from build123d import *

# Parameters (mm, degrees)
EXTRUDE_1_DEPTH     = 1300
SKETCH_3_R          = 2
CUT_EXTRUDE_1_DEPTH = 1301.046633779
CUT_EXTRUDE_2_DEPTH = 1500
SKETCH_5_R          = 2
CUT_EXTRUDE_3_DEPTH = 1301.046633779


with BuildPart() as part:
    # 草图2 → 凸台-拉伸1 (new body)
    with BuildSketch(Plane.XY):
        with BuildLine():
            Line((-0.5, 8.5), (0.5, 8.5))
            ThreePointArc((0.5, 8.5), (2.621320344, 7.621320344), (3.5, 5.5))
            Line((3.5, 5.5), (3.5, -5.5))
            ThreePointArc((3.5, -5.5), (2.621320344, -7.621320344), (0.5, -8.5))
            Line((0.5, -8.5), (-0.5, -8.5))
            ThreePointArc((-0.5, -8.5), (-2.621320344, -7.621320344), (-3.5, -5.5))
            Line((-3.5, -5.5), (-3.5, 5.5))
            ThreePointArc((-3.5, 5.5), (-2.621320344, 7.621320344), (-0.5, 8.5))
        make_face()
    extrude(amount=EXTRUDE_1_DEPTH)

    # 草图3 → 切除-拉伸1 (cut, through all)
    with BuildSketch(Plane.ZY.offset(3.5)):
        with Locations((100, 0)):
            Circle(SKETCH_3_R)
        with Locations((200, 0)):
            Circle(SKETCH_3_R)
        with Locations((300, 0)):
            Circle(SKETCH_3_R)
        with Locations((400, 0)):
            Circle(SKETCH_3_R)
        with Locations((500, 0)):
            Circle(SKETCH_3_R)
        with Locations((600, 0)):
            Circle(SKETCH_3_R)
        with Locations((700, 0)):
            Circle(SKETCH_3_R)
        with Locations((800, 0)):
            Circle(SKETCH_3_R)
        with Locations((900, 0)):
            Circle(SKETCH_3_R)
        with Locations((1000, 0)):
            Circle(SKETCH_3_R)
    extrude(amount=-CUT_EXTRUDE_1_DEPTH, mode=Mode.SUBTRACT)

    # 草图4 → 切除-拉伸2 (cut)
    with BuildSketch(Plane(origin=(0, 0, 0), x_dir=(-1, 0, 0), z_dir=(0, 0, -1))):
        with BuildLine():
            Line((-0.5, 7), (0.5, 7))
            ThreePointArc((0.5, 7), (1.560660172, 6.560660172), (2, 5.5))
            Line((2, 5.5), (2, -5.90279402))
            ThreePointArc((2, -5.90279402), (1.678635809, -6.678635809), (0.90279402, -7))
            Line((0.90279402, -7), (-0.90279402, -7))
            ThreePointArc((-0.90279402, -7), (-1.678635809, -6.678635809), (-2, -5.90279402))
            Line((-2, -5.90279402), (-2, 5.5))
            ThreePointArc((-2, 5.5), (-1.560660172, 6.560660172), (-0.5, 7))
        make_face()
    extrude(amount=-CUT_EXTRUDE_2_DEPTH, mode=Mode.SUBTRACT)

    # 草图5 → 切除-拉伸3 (cut, through all)
    with BuildSketch(Plane.ZY.offset(3.5)):
        with Locations((1100, 0)):
            Circle(SKETCH_5_R)
        with Locations((1200, 0)):
            Circle(SKETCH_5_R)
        with Locations((1250, 0)):
            Circle(SKETCH_5_R)
        with Locations((1150, 0)):
            Circle(SKETCH_5_R)
    extrude(amount=-CUT_EXTRUDE_3_DEPTH, mode=Mode.SUBTRACT)


solid = part.part
Input: part model. Units: mm. Frame: model coordinates. Give positions to 0.01 mm unless a question says otherwise; leave off trailing zeros. Order: outer loops, then holes, each group sorted by start corner. A loop starts at its lowest first (then second) coordinate and runs counter-clockwise, first axis right, second up. Notation, with made-up numbers: (-35, 33) - (-28, 33) arc R21 ccw to (-28, 45) - close; hole circle Ø3 at (41.5, 56). An arc over 180 degrees is marked (long way). Answer as a JSON object with one key per item and string values. Group by question number.
Q1. Line query: probe 1 along Y at (x, z) = (-3, 600); probe 2 along X at (y, z) = (-4, 558); probe 3 along Y at (x, z) = (1, 1101). Output: solid intervals per line, ascending.
Q2. Cut plane A-A, the plane z = 82. Output: boundary loops of the cut face in (x, y).
Q3. First-contact query: pin 1 Ø1 at (x, z) = (1.5, 350) entering from +Y; pin 2 Ø2 at (x, z) = (-2.5, 439) entering from +Y. Flat tips, straight axial feed; report the tip coordinate or a pass-through.
Results:
{
 "1": {"probe 1": "-7.16 to -2, 2 to 7.16", "probe 2": "-3.5 to -2, 2 to 3.5", "probe 3": "-8.46 to -7, 6.91 to 8.46"},
 "2": {"outline": "(-3.5, -5.5) arc R3 ccw to (-0.5, -8.5) - (0.5, -8.5) arc R3 ccw to (3.5, -5.5) - (3.5, 5.5) arc R3 ccw to (0.5, 8.5) - (-0.5, 8.5) arc R3 ccw to (-3.5, 5.5) - close; hole (-2, -5.9) arc R1.1 ccw to (-0.9, -7) - (0.9, -7) arc R1.1 ccw to (2, -5.9) - (2, 5.5) arc R1.5 ccw to (0.5, 7) - (-0.5, 7) arc R1.5 ccw to (-2, 5.5) - close"},
 "3": {"pin 1": "y = 8.46", "pin 2": "y = 8.33"}
}
